For this review, take the finished solid that the model builds, in its own axes (mm). A direction names the side the tool comes from. Round coordinates to 2 decimals unless told otherwise and drop trailing zeros. Order: outer loops, then holes, each group sorted by start corner. A loop starts at its lowest first (then second) coordinate and runs counter-clockwise, first axis right, second up. Notation, with made-up numbers: M -16,86 L 20,86 A25 cw 20,117 Z; hole C 88,-24 d11. An arc over 180 degrees is marked long. Answer as a JSON object with one key per item and string values.
from build123d import *

# Parameters (mm, degrees)
BOSS_EXTRUDE1_DEPTH  = 7
SKETCH6_R            = 2.25
CUT_EXTRUDE4_DEPTH   = 25
BOSS_EXTRUDE2_START  = -21
BOSS_EXTRUDE2_DEPTH  = 43
CUT_EXTRUDE5_DEPTH   = 28
FILLET1_R            = 15
FILLET1_OF_MIRROR1_R = 15
SKETCH12_W           = 7
SKETCH12_H           = 100
CUT_EXTRUDE6_DEPTH   = 24.5
SKETCH13_R           = 1.9
CUT_EXTRUDE7_DEPTH   = 24.5
SKETCH14_R           = 1.9
CUT_EXTRUDE8_DEPTH   = 7


with BuildPart() as part:
    # Sketch2 → Boss-Extrude1 (new body)
    with BuildSketch(Plane.XY):
        with BuildLine():
            Line((15, -200), (25, 0))
            ThreePointArc((25, 0), (0, 25), (-25, 0))
            Line((-25, 0), (-15, -200))
            ThreePointArc((-15, -200), (0, -215), (15, -200))
        make_face()
    extrude(amount=BOSS_EXTRUDE1_DEPTH)

    # Sketch6 → Cut-Extrude4 (cut)
    with BuildSketch(Plane.XY.offset(7)):
        with Locations((0, -200)):
            Circle(SKETCH6_R)
    extrude(amount=-CUT_EXTRUDE4_DEPTH, mode=Mode.SUBTRACT)

    # Sketch9 → Boss-Extrude2 (add)
    with BuildSketch(Plane.ZY.offset(BOSS_EXTRUDE2_START)):
        Polygon((0, -200), (0, -215), (-5, -215), (-5, -140), (0, -100), align=None)
    boss_extrude2 = extrude(amount=BOSS_EXTRUDE2_DEPTH)

    # Sketch10 → Cut-Extrude5 (cut, symmetric)
    with BuildSketch(Plane.XY.offset(7)):
        with BuildLine():
            Line((21, -100), (20, -100))
            Line((20, -100), (15, -200))
            ThreePointArc((15, -200), (10.606601767, -210.606601669), (1.38e-07, -215))
            Line((1.38e-07, -215), (21, -215))
            Line((21, -215), (21, -100))
        make_face()
        with BuildLine():
            Line((-22, -215), (1.38e-07, -215))
            ThreePointArc((1.38e-07, -215), (-10.606601669, -210.606601767), (-15, -200))
            Line((-15, -200), (-20, -100))
            Line((-20, -100), (-22, -100))
            Line((-22, -100), (-22, -215))
        make_face()
    cut_extrude5 = extrude(amount=CUT_EXTRUDE5_DEPTH, both=True, mode=Mode.SUBTRACT)

    # Fillet1
    fillet1_edges = [part.edges().sort_by_distance(p)[0] for p in [
        (0, -140, -5),
    ]]
    fillet(fillet1_edges, radius=FILLET1_R)

    # Mirror1: Boss-Extrude2 across plane
    add(boss_extrude2.mirror(Plane.XY.offset(3.5)))

    # Fillet1 of Mirror1
    fillet1_of_mirror1_edges = [part.edges().sort_by_distance(p)[0] for p in [
        (0, -140, 12),
    ]]
    fillet(fillet1_of_mirror1_edges, radius=FILLET1_OF_MIRROR1_R)

    # Mirror2: Cut-Extrude5 across plane
    add(cut_extrude5.mirror(Plane.XY.offset(3.5)), mode=Mode.SUBTRACT)

    # Sketch12 → Cut-Extrude6 (cut, symmetric)
    with BuildSketch(Plane.ZY):
        with Locations((3.5, -165)):
            Rectangle(SKETCH12_W, SKETCH12_H)
    extrude(amount=CUT_EXTRUDE6_DEPTH, both=True, mode=Mode.SUBTRACT)

    # Sketch13 → Cut-Extrude7 (cut, symmetric)
    with BuildSketch(Plane(origin=(0, 0, -5), x_dir=(-1, 0, 0), z_dir=(0, 0, -1))):
        with Locations(Location((0, -200, 0), (0, 0, 90))):
            Circle(SKETCH13_R)
    extrude(amount=CUT_EXTRUDE7_DEPTH, both=True, mode=Mode.SUBTRACT)

    # Sketch14 → Cut-Extrude8 (cut)
    with BuildSketch(Plane(origin=(0, 0, 0), x_dir=(-1, 0, 0), z_dir=(0, 0, -1))):
        Circle(SKETCH14_R)
    extrude(amount=-CUT_EXTRUDE8_DEPTH, mode=Mode.SUBTRACT)


solid = part.part
1) Add section A-A on y = -123. State the section outline as (x, z) points (3 decimals).
Geometry check:
{"outline": "M -18.85,-2.875 L 18.85,-2.875 L 18.85,0 L -18.85,0 Z; M -18.85,7 L 18.85,7 L 18.85,9.875 L -18.85,9.875 Z"}
2) Insertion check: P1, Ø5, axis at x = -13.5, z = -1.5, coming from the +Y side; P2, Ø1, axis at y = -38, z = 3, coming from the -X side (3 decimals); P3, Ø10, axis at y = -132, z = 3, coming from the -X side; P4, Ø3, axis at x = 0, y = -200, coming from the +Z side. Each pin has a flat end and moves straight along its axis. Give the tip position at first contact, or say it passes through.
Geometry check:
{"P1": "stops at y = 22.2", "P2": "stops at x = -23.125", "P3": "stops at x = -18.6", "P4": "passes through"}
3) Add section D-D on x = -11. State the section outline as (y, z) points.
Geometry check:
{"outline": "M -210.2,-5 L -140.93,-5 A15 ccw -139.07,-4.88 L -100,0 L 22.45,0 L 22.45,7 L -100,7 L -139.07,11.88 A15 ccw -140.93,12 L -210.2,12 L -210.2,7 L -115,7 L -115,0 L -210.2,0 Z"}
4) Machinability: for faces 4 (the flat face through (0, -166, 0)), 5 (the flat face through (18.96, -120.82, 7.16)), 6 (the flat face through (0, -37, 7)), which of the approach directions +Z, -Z, +X, -X, +Y, -Y give a long, thin tool a straight path to every point of the face, cutting with its end or side? Answer none if there is none.
Geometry check:
{"face 4": "+X, -X, -Y", "face 5": "+Z, -Z, +X, -Y", "face 6": "+Z, +X, -X, +Y"}
5) Add section B-B on x = 10. State the section outline as (y, z) points.
Geometry check:
{"outline": "M -211.18,-5 L -140.93,-5 A15 ccw -139.07,-4.88 L -100,0 L 22.91,0 L 22.91,7 L -100,7 L -139.07,11.88 A15 ccw -140.93,12 L -211.18,12 L -211.18,7 L -115,7 L -115,0 L -211.18,0 Z"}
6) Add section C-C on y = -68. State the section outline as (x, z) points.
Geometry check:
{"outline": "M -21.6,0 L 21.6,0 L 21.6,7 L -21.6,7 Z"}
7) Mouldability with a two-part tool opening along Z and no side actions: class faces 1 (the flat face through (0, -178, 12)), 2 (the flat face through (0, -166, 7)), 3 (the flat face through (0, -37, 0)) as +Z half, -Z half, draft (parallel to the pull), parting line (faces both ways), or undercut.
Geometry check:
{"face 1": "+Z half", "face 2": "undercut", "face 3": "-Z half"}
8) For L1, parallel to Y at x = 0, z = 5; L2, parallel to X at y = -200, z = -2.8; L3, parallel to Z at x = -5, y = -168, list the stretches that pass through material, from the lowest coordinate up.
Geometry check:
{"L1": "y = -115 to -1.9, 1.9 to 25", "L2": "x = -15 to -1.9, 1.9 to 15", "L3": "z = -5 to 0, 7 to 12"}
